```python
from build123d import *

# Parameters (mm, degrees)
F1_DEPTH = 7.2
F2_W     = 3.6
F2_H     = 2.4
F3_DEPTH = 7.201
F5_DEPTH = 6.5
F6_W     = 7
F6_H     = 0.7
F7_DEPTH = 7.201
F8_R     = 0.25
F9_R     = 0.1


with BuildPart() as f1:
    # F0 (on Front) → F1 (new body)
    with BuildSketch(Plane.XZ):
        Polygon((-3.5, 6.35), (-3.5, 1.1), (3.5, 1.1), (3.5, 6.35), (1.87, 7.9), (-1.87, 7.9), align=None)
    extrude(amount=F1_DEPTH)

    # F2 (on face) → F3 (cut, through all)
    with BuildSketch(Plane.XZ.offset(7.2)):
        with Locations((0, 2.3)):
            Rectangle(F2_W, F2_H)
    extrude(amount=-F3_DEPTH, mode=Mode.SUBTRACT)

    # F4 (on face) → F5 (cut)
    with BuildSketch(Plane(origin=(0, 0, 0), x_dir=(-1, 0, 0), z_dir=(0, 1, 0))):
        Polygon((-2.75, 1.1), (2.75, 1.1), (2.75, 6.028231), (1.570333, 7.15), (-1.570333, 7.15), (-2.75, 6.028231), align=None)
    extrude(amount=-F5_DEPTH, mode=Mode.SUBTRACT)

    # F6 (on face) → F7 (cut, through all)
    with BuildSketch(Plane.XZ.offset(7.2)):
        with Locations((0, 1.45)):
            Rectangle(F6_W, F6_H)
    extrude(amount=-F7_DEPTH, mode=Mode.SUBTRACT)

    # F8
    f8_edges = [f1.edges().sort_by_distance(p)[0] for p in [
        (-3.5, -3.6, 6.35),
        (-1.87, -3.6, 7.9),
        (1.87, -3.6, 7.9),
        (3.5, -3.6, 6.35),
    ]]
    fillet(f8_edges, radius=F8_R)

    # F9
    f9_edges = [f1.edges().sort_by_distance(p)[0] for p in [
        (-3.5, -7.2, 4.021372),
    ]]
    fillet(f9_edges, radius=F9_R)


solid = f1.part
```
Here's how the part is built. I have some questions about the finished solid (model axes, mm). A direction names the side the tool comes from. Round coordinates to 2 decimals unless told otherwise and drop trailing zeros. Write each loop counter-clockwise with the first axis right and the second up, starting at its lowest first coordinate (ties: lowest second). Pieces come first, ordered by that corner, then holes. Notation, with made-up numbers: M 8.25,28.25 L 64.25,28.25 A24 cw 64.25,63.25 Z; hole C 74,85.25 d7. An arc over 180 degrees is marked long. Answer as CSV lines item,"result". Start each with the question number.
1. On a 3-axis mill with a long thin cutter (end or side, diameter ignored), from which of +Z, -Z, +X, -X, +Y, -Y can I reach the whole of each face in a straight line? I mean faces 4 (the flat face through (-2.17, -3.2, 6.58)), 5 (the flat face through (0, -4, 7.9)). Say none if no direction works.
2. Suppose I cut it at B-B on y = -2.75. Write out the boundary of the cut face in (x, z).
3. Suppose I cut it at C-C on x = 0.5. Write out the boundary of the cut face in (y, z).
4. I'm going to push flat-ended pins straight in: pin 1 Ø1 at (x, y) = (-2.5, -5.5) entering from +Z; pin 2 Ø3.5 at (x, y) = (0, -3) entering from -Z; pin 3 Ø1 at (x, y) = (0, -4) entering from -Z. Where does each tip first touch, or does it pass through?
5. Suppose I cut it at A-A on z = 2.5. Write out the boundary of the cut face in (x, y).
6. Thinking about a two-plate mould opening in X: for faces 1 (the flat face through (2.69, -3.5, 7.12)), 2 (the flat face through (-0.28, 0, 7.35)), 3 (the flat face through (-2.75, -3, 4)), which applies, released by +X, released by -X, zero draft, split by the parting line, or undercut?
7. I need wall thicknesses on probe 1 along X at (y, z) = (-4.5, 2.75); probe 2 along Y at (x, z) = (2, 4); probe 3 along Z at (x, y) = (-0.75, -2). Which ranges of each line are inside material? Lowest first, please.
8. Suppose I cut it at D-D on z = 5. Write out the boundary of the cut face in (x, y).
Check result:
1,face 4,"-Z, +Y"
1,face 5,"+Z, +X, -X, +Y, -Y"
2,outline,"M -3.5,1.8 L -2.75,1.8 L -2.75,6.03 L -1.57,7.15 L 1.57,7.15 L 2.75,6.03 L 2.75,1.8 L 3.5,1.8 L 3.5,6.24 A0.25 ccw 3.42,6.42 L 1.94,7.83 A0.25 ccw 1.77,7.9 L -1.77,7.9 A0.25 ccw -1.94,7.83 L -3.42,6.42 A0.25 ccw -3.5,6.24 Z"
3,outline,"M -7.2,3.5 L -6.5,3.5 L -6.5,7.15 L 0,7.15 L 0,7.9 L -7.1,7.9 A0.1 ccw -7.2,7.8 Z"
4,pin 1,"stops at z = 7.78"
4,pin 2,"stops at z = 6.98"
4,pin 3,"stops at z = 7.15"
5,outline,"M -3.5,-7.1 A0.1 ccw -3.4,-7.2 L -1.8,-7.2 L -1.8,-6.5 L -2.75,-6.5 L -2.75,0 L -3.5,0 Z; M 1.8,-7.2 L 3.4,-7.2 A0.1 ccw 3.5,-7.1 L 3.5,0 L 2.75,0 L 2.75,-6.5 L 1.8,-6.5 Z"
6,face 1,"released by +X"
6,face 2,"zero draft"
6,face 3,"undercut"
7,probe 1,"x = -3.5 to -2.75, 2.75 to 3.5"
7,probe 2,"y = -7.2 to -6.5"
7,probe 3,"z = 7.15 to 7.9"
8,outline,"M -3.5,-7.1 A0.1 ccw -3.4,-7.2 L 3.4,-7.2 A0.1 ccw 3.5,-7.1 L 3.5,0 L 2.75,0 L 2.75,-6.5 L -2.75,-6.5 L -2.75,0 L -3.5,0 Z"
